from build123d import *

# Parameters (mm, degrees)
SKETCH_1_W              = 27
SKETCH_1_H              = 21.7
EXTRUDE_1_DEPTH         = 10
SKETCH_2_W              = 26
SKETCH_2_H              = 9.5
EXTRUDE_2_DEPTH         = 6.5
SKETCH_3_W              = 26
SKETCH_3_H              = 9.5
EXTRUDE_3_DEPTH         = 6.5
CUT_EXTRUDE_1_DEPTH     = 38.567805366
DRAFT_1_ANGLE           = 23.473307954
HOLE_WIZARD_3_3_3_3_1_D = 3.3


with BuildPart() as part:
    # 草图1 → 凸台-拉伸1 (new body)
    with BuildSketch(Plane.XZ.offset(5)):
        Rectangle(SKETCH_1_W, SKETCH_1_H)
    extrude(amount=-EXTRUDE_1_DEPTH)

    # 草图2 → 凸台-拉伸2 (add)
    with BuildSketch(Plane.XY.offset(10.85)):
        with Locations((0, -0.25)):
            Rectangle(SKETCH_2_W, SKETCH_2_H)
    extrude(amount=EXTRUDE_2_DEPTH)

    # 草图3 → 凸台-拉伸3 (add)
    with BuildSketch(Plane(origin=(0, 0, -10.85), x_dir=(-1, 0, 0), z_dir=(0, 0, -1))):
        with Locations((0, -0.25)):
            Rectangle(SKETCH_3_W, SKETCH_3_H)
    extrude(amount=EXTRUDE_3_DEPTH)

    # 草图4 → 切除-拉伸1 (cut, through all)
    with BuildSketch(Plane.XY.offset(17.35)):
        Polygon((6, -5), (3, -4), (4, -3.565741454), (4, 0), (-4, 0), (-4, -3.565741454), (-3, -4), (-6, -5), align=None)
    extrude(amount=-CUT_EXTRUDE_1_DEPTH, mode=Mode.SUBTRACT)

    # 拔模1
    draft_1_faces = [part.faces().sort_by_distance(p)[0] for p in [
        (-4, -1.782870727, 0),
        (4, -1.782870727, 0),
    ]]
    draft(draft_1_faces, Plane(origin=(4, 0, -17.35), x_dir=(-1, 0, 0), z_dir=(0, -1, 0)), DRAFT_1_ANGLE)

    # Ø3.3 (3.3) 直径孔1 (through all)
    with Locations(Plane(origin=(0, 5, 0), x_dir=(1, 0, 0), z_dir=(0, 1, 0))):
        with Locations((10, -7.5), (-10, -7.5), (-10, 7.5), (10, 7.5)):
            Hole(HOLE_WIZARD_3_3_3_3_1_D / 2)


solid = part.part
Can you work these out from the model? Positions are in its coordinate system, mm. A direction names the side the tool comes from. Give positions to 0.01 mm unless a question says otherwise; leave off trailing zeros. Write each loop counter-clockwise with the first axis right and the second up, starting at its lowest first coordinate (ties: lowest second). Pieces come first, ordered by that corner, then holes. Notation, with made-up numbers: (8.25, -15) -> (39.25, -15) arc R36 ccw to (39.25, 19) -> close; hole circle Ø8 at (89, 20). An arc over 180 degrees is marked (long way). Answer as a JSON object with one key per item and string values. Group by question number.
Item 1: We'd pull the mould along Y, two halves only. Please class faces 6 (the face through (-6.1, 4.8, -10.85)), 7 (the face through (10, -5, 0)), 8 (the face through (0, 0, 0)), 9 (the face through (0, 5, 0)): +Y half, -Y half, draft (parallel to the pull), parting line (faces both ways), or undercut.
Item 2: I'm going to push flat-ended pins straight in: P1, Ø3.5, axis at x = 3.5, z = -13.5, coming from the +Y side; P2, Ø3.5, axis at y = 0, z = 14, coming from the +X side; P3, Ø1.5, axis at x = 3.5, z = -7.5, coming from the -Y side. Where does each tip first touch, or does it pass through?
Item 3: Suppose I cut it at C-C (x = 10). Please give me the cut outline in (y, z), plus the area to 4 significant figures.
Item 4: For faces 1 (the face through (-13, 0, 14)), 2 (the face through (-4.17, -3.49, 0.24)), 3 (the face through (-4.5, -4.5, 0.2)), 4 (the face through (0, 1, 17.35)), 5 (the face through (0, 4.5, 14)), which set-ups out of +Z, -Z, +X, -X, +Y, -Y let a thin tool reach every point of the face, with its end or its side?
Item 5: Suppose I cut it at D-D (x = 4.5). Please give me the cut outline in (y, z).
Item 6: Suppose I cut it at A-A (y = -0.5). Please give me the cut outline in (x, z).
Item 7: Suppose I cut it at B-B (z = 7). Please give me the cut outline in (x, y).
Item 8: Please list where these lines run through material, in increasing order: line 1 (X direction, y = 0.25, z = 7.5); line 2 (Z direction, x = -10, y = 0.75); line 3 (Z direction, x = 9.25, y = -2). Write a range as [from, to].
Findings:
{
 "1": {"face 6": "draft", "face 7": "-Y half", "face 8": "undercut", "face 9": "+Y half"},
 "2": {"P1": "stops at y = 4.5", "P2": "stops at x = 13", "P3": "stops at y = -4.42"},
 "3": {"outline": "(-5, -17.35) -> (4.5, -17.35) -> (4.5, -10.85) -> (5, -10.85) -> (5, -9.15) -> (-5, -9.15) -> close; (-5, -5.85) -> (5, -5.85) -> (5, 5.85) -> (-5, 5.85) -> close; (-5, 9.15) -> (5, 9.15) -> (5, 10.85) -> (4.5, 10.85) -> (4.5, 17.35) -> (-5, 17.35) -> close", "area": "274.5 mm²"},
 "4": {"face 1": "+Z, -X, +Y, -Y", "face 2": "+Z, -Z", "face 3": "+Z, -Z, -Y", "face 4": "+Z, +X, -X, +Y, -Y", "face 5": "+Z, +X, -X, +Y"},
 "5": {"outline": "(-4.5, -17.35) -> (-3.35, -17.35) -> (-3.35, 17.35) -> (-4.5, 17.35) -> close; (-1.15, -17.35) -> (4.5, -17.35) -> (4.5, -10.85) -> (5, -10.85) -> (5, 10.85) -> (4.5, 10.85) -> (4.5, 17.35) -> (-1.15, 17.35) -> close"},
 "6": {"outline": "(-13.5, -10.85) -> (-13, -10.85) -> (-13, -17.35) -> (-4.22, -17.35) -> (-4.22, 17.35) -> (-13, 17.35) -> (-13, 10.85) -> (-13.5, 10.85) -> close; (4.22, -17.35) -> (13, -17.35) -> (13, -10.85) -> (13.5, -10.85) -> (13.5, 10.85) -> (13, 10.85) -> (13, 17.35) -> (4.22, 17.35) -> close; hole circle Ø3.3 at (-10, -7.5); hole circle Ø3.3 at (-10, 7.5); hole circle Ø3.3 at (10, -7.5); hole circle Ø3.3 at (10, 7.5)"},
 "7": {"outline": "(-13.5, -5) -> (-11.57, -5) -> (-11.57, 5) -> (-13.5, 5) -> close; (-8.43, -5) -> (-6, -5) -> (-3, -4) -> (-5.3, -3) -> (-4, 0) -> (4, 0) -> (5.3, -3) -> (3, -4) -> (6, -5) -> (8.43, -5) -> (8.43, 5) -> (-8.43, 5) -> close; (11.57, -5) -> (13.5, -5) -> (13.5, 5) -> (11.57, 5) -> close"},
 "8": {"line 1": "x = [-13.5, -11.65], [-8.35, 8.35], [11.65, 13.5]", "line 2": "z = [-17.35, -9.15], [-5.85, 5.85], [9.15, 17.35]", "line 3": "z = [-17.35, -8.97], [-6.03, 6.03], [8.97, 17.35]"}
}
